Input: part model. Units: mm. Frame: model coordinates. Face numbers are marked on the shaded views. A direction names the side the tool comes from. Round coordinates to 2 decimals unless told otherwise and drop trailing zeros. Write each loop counter-clockwise with the first axis right and the second up, starting at its lowest first coordinate (ties: lowest second). Pieces come first, ordered by that corner, then holes. Notation, with made-up numbers: M -8,74 L 3,74 A33 cw 3,111 Z; hole C 32.5,11.25 d1. An arc over 180 degrees is marked long. Answer as CSV lines item,"result". Start each with the question number.
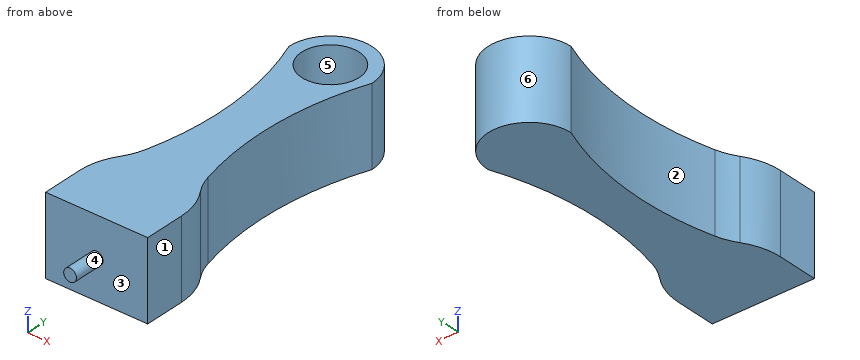
Autodesk Inventor part; units mm, degrees
ref_plane "YZ Plane" through (0, 0, 0) normal (1, 0, 0) x (0, 1, 0)
ref_plane "XZ Plane" through (0, 0, 0) normal (0, 1, 0) x (-1, 0, 0)
ref_plane "XY Plane" through (0, 0, 0) normal (0, 0, 1) x (1, 0, 0)
sketch "Sketch1" plane through (0, 0, 0) normal (0, 1, 0) x (-1, 0, 0)
  line L0 (0, 0) -> (16, 0)
  line L1 (16, 0) -> (16, -12.3)
  line L2 (16, -12.3) -> (0, -12.3)
  line L3 (0, -12.3) -> (0, 0)
  dimension "d0" = 16
  dimension "d1" = 12.3
extrude "Extrusion1" add sketch "Sketch1" along normal blind 10
sketch "Sketch2" plane through (0, 10, 0) normal (0, 1, 0) x (1, 0, 0)
  line L0 (-16, 0) -> (0, 0)
  line L1 (-8, 0) -> (-8, 12.3)
  line L2 (0, 12.3) -> (-16, 12.3)
  line L3 (-14.5, 0) -> (-14.5, 12.3)
  line L4 (-1.5, 0) -> (-1.5, 12.3)
  dimension "d4" = 6.5
  dimension "d5" = 6.5
extrude "Extrusion2" add sketch "Sketch2" along normal blind 40.5
sketch "Sketch3" plane through (-16, 0, 0) normal (0, 0, 1) x (1, 0, 0)
  line L0 (14.5, 50.5) -> (1.5, 50.5)
  line L1 (8, 50.5) -> (8, 0)
  line L2 (0, 0) -> (16, 0)
  circle A0 centre (8, 44) radius 4.5
  line L3 (1.5, 50.5) -> (14.5, 50.5)
  circle A1 centre (8, 44) radius 6.5
  line L4 (14.5, 10) -> (14.5, 50.5)
  line L5 (14.5, 30.25) -> (1.5, 30.25)
  line L6 (1.5, 10) -> (1.5, 50.5)
  line L7 (8, 30.25) -> (11.5, 30.25)
  arc A2 (14.5, 44) -> (14.5, 10) centre (59.4062, 27) ccw
  line L8 (8, 30.25) -> (4.5, 30.25)
  arc A3 (1.5, 10) -> (1.5, 44) centre (-43.4062, 27) ccw
  dimension "d8" = 6.5
  dimension "d9" = 9
  dimension "d10" = 13
  dimension "d11" = 3.5
  dimension "d12" = 3.5
extrude "Extrusion3" cut sketch "Sketch3" against normal blind 13.5 contours L4 A1 L0 | A1 L6 L0 | L4 L5 A2 A1 | A1 A2 | A3 A1 | A1 A3 L5 L6 | L4 A2 L5 | L5 A3 L6
fillet "Fillet1" radius 10 4 edges at (0, 10, -6.15) (-1.5, 10, -6.15) (-14.5, 10, -6.15) (-16, 10, -6.15)
sketch "Sketch4" plane through (-16, 0, 0) normal (0, 0, 1) x (1, 0, 0)
  arc A0 (14.5, 44) -> (1.5, 44) centre (8, 44) ccw
  circle A1 centre (8, 44) radius 4.5
  point P0 (16, 0)
  dimension "d16" = 9
extrude "Extrusion4" cut sketch "Sketch4" against normal blind 8.23
sketch "Sketch5" plane through (0, 0, 0) normal (0, -1, 0) x (1, 0, 0)
  line L0 (-16, 0) -> (0, 0)
  line L1 (-8, 0) -> (-8, -12.3)
  line L2 (0, -12.3) -> (-16, -12.3)
  circle A0 centre (-8, -6.15) radius 1
extrude "Extrusion5" add sketch "Sketch5" along normal blind 5
properties part number "pawn"
Item 1: Cut plane A-A, the plane z = -1.25. Return loops of the section in (x, y), plus the area to 3 significant figures.
Item 2: Pin query (flat end, axial travel): pin 1 Ø3.5 at (x, z) = (-5.5, -5.5) entering from -Y; pin 2 Ø6 at (y, z) = (33, -9.5) entering from +X; pin 3 Ø6 at (y, z) = (33, -9) entering from -X; pin 4 Ø1 at (y, z) = (23, -5.5) entering from -X. Return the tip coordinate at first contact, or that it passes through.
Item 3: Cut plane B-B, the plane x = -8. Return loops of the section in (y, z), plus the area to 3 significant figures.
Item 4: Draft query along Y for the marked faces 1, 2 and 3. Return one class per face: +Y half, -Y half, draft (parallel to the pull), parting line (faces both ways), or undercut.
Item 5: Cut plane D-D, the plane z = -6.15. Return loops of the section in (x, y), plus the area to 3 significant figures.
Item 6: Line query: line 1 (Y direction, x = -8, z = -6); line 2 (Y direction, x = -8, z = -2.25); line 3 (X direction, y = 44, z = -10.25). Output: solid intervals per line, ascending. Write a range as [from, to].
Item 7: Access query for the marked faces 4, 5 and 6. Directions: +Z, -Z, +X, -X, +Y, -Y. A direction counts if a zero-diameter tool reaches every point of the face in a straight line with its end or side. Return the directions, or none.
Item 8: Cut plane C-C, the plane z = -9. Return loops of the section in (x, y), plus the area to 3 significant figures.
Results list:
1,outline,"M -16,0 L 0,0 L 0,6.35 A10 ccw -1.7,11.94 A10 cw -3.09,15.03 A48.02 cw -1.5,44 A6.5 ccw -14.5,44 A48.02 cw -12.91,15.03 A10 cw -14.3,11.94 A10 ccw -16,6.35 Z; hole C -8,44 d9"
1,area,"465 mm²"
2,pin 1,"y = -5"
2,pin 2,"x = -3.76"
2,pin 3,"x = -12.24"
2,pin 4,"x = -11.6"
3,outline,"M -5,-7.15 L 0,-7.15 L 0,-12.3 L 50.5,-12.3 L 50.5,0 L 48.5,0 L 48.5,-8.23 L 39.5,-8.23 L 39.5,0 L 0,0 L 0,-5.15 L -5,-5.15 Z"
3,area,"557 mm²"
4,face 1,"draft"
4,face 2,"undercut"
4,face 3,"-Y half"
5,outline,"M -16,0 L -9,0 L -9,-5 L -7,-5 L -7,0 L 0,0 L 0,6.35 A10 ccw -1.7,11.94 A10 cw -3.09,15.03 A48.02 cw -1.5,44 A6.5 ccw -14.5,44 A48.02 cw -12.91,15.03 A10 cw -14.3,11.94 A10 ccw -16,6.35 Z; hole C -8,44 d9"
5,area,"475 mm²"
6,line 1,"[-5, 39.5], [48.5, 50.5]"
6,line 2,"[0, 39.5], [48.5, 50.5]"
6,line 3,"[-14.5, -1.5]"
7,face 4,"-Y"
7,face 5,"+Z"
7,face 6,"+Z, -Z, +Y"
8,outline,"M -16,0 L 0,0 L 0,6.35 A10 ccw -1.7,11.94 A10 cw -3.09,15.03 A48.02 cw -1.5,44 A6.5 ccw -14.5,44 A48.02 cw -12.91,15.03 A10 cw -14.3,11.94 A10 ccw -16,6.35 Z"
8,area,"528 mm²"
